Design review of the part built by this model. Coordinates are the model's own, in mm. A direction names the side the tool comes from. Coordinates: 2 decimals unless noted, no trailing zeros. Write each loop counter-clockwise with the first axis right and the second up, starting at its lowest first coordinate (ties: lowest second). Pieces come first, ordered by that corner, then holes.
Q1. Take a section at A-A (x = -18.5). Give the boundary of the cut face in (y, z), and give its area (3 significant figures).
Q2. Machinability: for faces 1 (the flat face through (-137.09, 3.13, 355.27)), 2 (the flat face through (-211.102, 3.131, -68.679)), 3 (the cylindrical face through (-120.638, 3.219, 125.96)), 4 (the flat face through (-138.21, 3.13, -107.53)), which of the approach directions +Z, -Z, +X, -X, +Y, -Y give a long, thin tool a straight path to every point of the face, cutting with its end or side? Answer none if there is none.
Q3. Insertion check: pin 1 (1.5 mm diameter, centred on y = 3, z = 326.5, fed in from -X); pin 2 (1 mm diameter, centred on y = 1.5, z = 330, fed in from +X); pin 3 (1.5 mm diameter, centred on x = 63.5, y = 4.5, fed in from +Z). Each pin has a flat end and moves straight along its axis. Give the tip position at first contact, or say it passes through.
Q4. Take a section at C-C (y = 3.75). State how many separate pieces and enclosed holes the cut face has, and give its area (3 significant figures).
Q5. For probe 1 along Z at (x, y) = (230, 2.75); probe 2 along Z at (x, y) = (-36, 5); probe 3 along Z at (x, y) = (159, 1), list the stretches that pass through material, from the lowest coordinate up.
Q6. Take a section at B-B (z = 196). Give the boundary of the cut face in (x, y).
Q7. Mouldability with a two-part tool opening along Z and no side actions: class faces 5 (the cylindrical face through (107.938, 3.219, 123.726)), 6 (the flat face through (-223.304, 3.131, -171.742)), 7 (the flat face through (138.213, 3.131, 357.218)) as pulls with the +Z half, pulls with the -Z half, needs draft (parallel to the pull), parting line crosses it, or undercut.
```python
from build123d import *

# Parameters (mm, degrees)
BOSS_EXTRUDE1_DEPTH     = 6.35
FILLET1_R               = 19.05
CUT_EXTRUDE1_DEPTH      = 503.879504709
SKETCH4_R               = 2.54
CUT_EXTRUDE2_DEPTH      = 503.879504709
SKETCH6_R               = 1.905
CUT_EXTRUDE3_DEPTH      = 503.879504709
MIRROR2_COPY_1_SKETCH_R = 2.54
MIRROR2_COPY_1_DEPTH    = 503.879504709
MIRROR2_COPY_2_SKETCH_R = 1.905
MIRROR2_COPY_2_DEPTH    = 503.879504709
FILLET2_R               = 12.7
SKETCH7_R               = 1.524
CUT_EXTRUDE4_DEPTH      = 503.879504709


with BuildPart() as part:
    # Sketch1 → Boss-Extrude1 (new body)
    with BuildSketch(Plane(origin=(0, 0, 0), x_dir=(1, 0, 0), z_dir=(0, 1, 0))):
        Polygon((-171.45, 0), (-258.780132361, 151.260226281), (-187.289735278, 192.535226281), (-92.039735278, 27.55738686), (92.039735278, 27.55738686), (187.289735278, 192.535226281), (258.780132361, 151.260226281), (171.45, 0), (171.45, -249.685226281), (258.780132361, -400.945452561), (187.289735278, -442.220452561), (92.039735278, -277.24261314), (-92.039735278, -277.24261314), (-187.289735278, -442.220452561), (-258.780132361, -400.945452561), (-171.45, -249.685226281), align=None)
    extrude(amount=BOSS_EXTRUDE1_DEPTH)

    # Fillet1
    fillet1_edges = [part.edges().sort_by_distance(p)[0] for p in [
        (-171.45, 3.175, 0),
        (-258.780132361, 3.175, -151.260226281),
        (-187.289735278, 3.175, -192.535226281),
        (-92.039735278, 3.175, -27.55738686),
        (92.039735278, 3.175, -27.55738686),
        (187.289735278, 3.175, -192.535226281),
        (258.780132361, 3.175, -151.260226281),
        (171.45, 3.175, 249.685226281),
        (258.780132361, 3.175, 400.945452561),
        (187.289735278, 3.175, 442.220452561),
        (92.039735278, 3.175, 277.24261314),
        (-92.039735278, 3.175, 277.24261314),
        (-187.289735278, 3.175, 442.220452561),
        (-258.780132361, 3.175, 400.945452561),
        (-171.45, 3.175, 249.685226281),
    ]]
    fillet(fillet1_edges, radius=FILLET1_R)

    # Sketch2 → Cut-Extrude1 (cut, through all)
    with BuildSketch(Plane(origin=(0, 6.35, 0), x_dir=(1, 0, 0), z_dir=(0, 1, 0))):
        with BuildLine():
            Line((-69.85, -74.04261314), (57.15, -74.04261314))
            ThreePointArc((57.15, -74.04261314), (107.95, -124.84261314), (57.15, -175.64261314))
            Line((57.15, -175.64261314), (-69.85, -175.64261314))
            ThreePointArc((-69.85, -175.64261314), (-120.65, -124.84261314), (-69.85, -74.04261314))
        make_face()
    cut_extrude1 = extrude(amount=-CUT_EXTRUDE1_DEPTH, mode=Mode.SUBTRACT)

    # Sketch4 → Cut-Extrude2 (cut, through all)
    with BuildSketch(Plane.XZ):
        with Locations(Location((198.392135104, -167.061146864, 0), (0, 0, 270))):
            Circle(SKETCH4_R)
        with Locations(Location((214.889919046, -157.536146864, 0), (0, 0, 270))):
            Circle(SKETCH4_R)
        with Locations(Location((231.387702988, -148.011146864, 0), (0, 0, 270))):
            Circle(SKETCH4_R)
        with Locations(Location((141.242135104, -68.074443212, 0), (0, 0, 90))):
            Circle(SKETCH4_R)
        with Locations(Location((174.237702988, -49.024443212, 0), (0, 0, 90))):
            Circle(SKETCH4_R)
        with Locations(Location((157.739919046, -58.549443212, 0), (0, 0, 90))):
            Circle(SKETCH4_R)
    cut_extrude2 = extrude(amount=-CUT_EXTRUDE2_DEPTH, mode=Mode.SUBTRACT)

    # Sketch6 → Cut-Extrude3 (cut, through all)
    with BuildSketch(Plane(origin=(0, 6.35, 0), x_dir=(1, 0, 0), z_dir=(0, 1, 0))):
        with Locations(Location((198.963220068, 100.740295038, 0), (0, 0, 270))):
            Circle(SKETCH6_R)
        with Locations(Location((185.951828097, 97.253903067, 0), (0, 0, 270))):
            Circle(SKETCH6_R)
        with Locations(Location((182.465436126, 110.265295038, 0), (0, 0, 270))):
            Circle(SKETCH6_R)
        with Locations(Location((195.476828097, 113.751687009, 0), (0, 0, 270))):
            Circle(SKETCH6_R)
    cut_extrude3 = extrude(amount=-CUT_EXTRUDE3_DEPTH, mode=Mode.SUBTRACT)

    # Mirror1: Cut-Extrude2, Cut-Extrude3 across plane
    add(cut_extrude2.mirror(Plane(origin=(0, 0, 0), x_dir=(0, 0, 1), z_dir=(1, 0, 0))), mode=Mode.SUBTRACT)
    add(cut_extrude3.mirror(Plane(origin=(0, 0, 0), x_dir=(0, 0, 1), z_dir=(1, 0, 0))), mode=Mode.SUBTRACT)

    # Mirror2: Cut-Extrude1, Cut-Extrude2, Cut-Extrude3 across plane
    add(cut_extrude1.mirror(Plane(origin=(0, 0, 124.84261314), x_dir=(1, 0, 0), z_dir=(0, 0, -1))), mode=Mode.SUBTRACT)
    add(cut_extrude2.mirror(Plane(origin=(0, 0, 124.84261314), x_dir=(1, 0, 0), z_dir=(0, 0, -1))), mode=Mode.SUBTRACT)
    add(cut_extrude3.mirror(Plane(origin=(0, 0, 124.84261314), x_dir=(1, 0, 0), z_dir=(0, 0, -1))), mode=Mode.SUBTRACT)

    # Mirror2 copy 1 sketch → Mirror2 copy 1 (cut, through all)
    with BuildSketch(Plane(origin=(0, 0, 249.685226281), x_dir=(-1, 0, 0), z_dir=(0, -1, 0))):
        with Locations(Location((198.392135104, -167.061146864, 0), (0, 0, 270))):
            Circle(MIRROR2_COPY_1_SKETCH_R)
        with Locations(Location((214.889919046, -157.536146864, 0), (0, 0, 270))):
            Circle(MIRROR2_COPY_1_SKETCH_R)
        with Locations(Location((231.387702988, -148.011146864, 0), (0, 0, 270))):
            Circle(MIRROR2_COPY_1_SKETCH_R)
        with Locations(Location((141.242135104, -68.074443212, 0), (0, 0, 90))):
            Circle(MIRROR2_COPY_1_SKETCH_R)
        with Locations(Location((174.237702988, -49.024443212, 0), (0, 0, 90))):
            Circle(MIRROR2_COPY_1_SKETCH_R)
        with Locations(Location((157.739919046, -58.549443212, 0), (0, 0, 90))):
            Circle(MIRROR2_COPY_1_SKETCH_R)
    extrude(amount=-MIRROR2_COPY_1_DEPTH, mode=Mode.SUBTRACT)

    # Mirror2 copy 2 sketch → Mirror2 copy 2 (cut, through all)
    with BuildSketch(Plane(origin=(0, 6.35, 249.685226281), x_dir=(-1, 0, 0), z_dir=(0, 1, 0))):
        with Locations(Location((198.963220068, 100.740295038, 0), (0, 0, 270))):
            Circle(MIRROR2_COPY_2_SKETCH_R)
        with Locations(Location((185.951828097, 97.253903067, 0), (0, 0, 270))):
            Circle(MIRROR2_COPY_2_SKETCH_R)
        with Locations(Location((182.465436126, 110.265295038, 0), (0, 0, 270))):
            Circle(MIRROR2_COPY_2_SKETCH_R)
        with Locations(Location((195.476828097, 113.751687009, 0), (0, 0, 270))):
            Circle(MIRROR2_COPY_2_SKETCH_R)
    extrude(amount=-MIRROR2_COPY_2_DEPTH, mode=Mode.SUBTRACT)

    # Fillet2
    fillet2_edges = [part.edges().sort_by_distance(p)[0] for p in [
        (171.45, 3.175, 0),
    ]]
    fillet(fillet2_edges, radius=FILLET2_R)

    # Sketch7 → Cut-Extrude4 (cut, through all)
    with BuildSketch(Plane(origin=(0, 6.35, 0), x_dir=(1, 0, 0), z_dir=(0, 1, 0))):
        with Locations(Location((-97.538996592, 14.85738686, 0), (0, 0, 270))):
            Circle(SKETCH7_R)
        with Locations(Location((-97.538996592, -6.73261314, 0), (0, 0, 270))):
            Circle(SKETCH7_R)
        with Locations(Location((-65.788996592, 14.85738686, 0), (0, 0, 270))):
            Circle(SKETCH7_R)
        with Locations(Location((-65.788996592, -6.73261314, 0), (0, 0, 270))):
            Circle(SKETCH7_R)
        with Locations(Location((97.538996592, -6.73261314, 0), (0, 0, 90))):
            Circle(SKETCH7_R)
        with Locations(Location((97.538996592, 14.85738686, 0), (0, 0, 90))):
            Circle(SKETCH7_R)
        with Locations(Location((65.788996592, 14.85738686, 0), (0, 0, 90))):
            Circle(SKETCH7_R)
        with Locations(Location((65.788996592, -6.73261314, 0), (0, 0, 90))):
            Circle(SKETCH7_R)
    extrude(amount=-CUT_EXTRUDE4_DEPTH, mode=Mode.SUBTRACT)


solid = part.part
```
Response:
1. outline: (0, -27.56) - (6.35, -27.56) - (6.35, 74.04) - (0, 74.04) - close; (0, 175.64) - (6.35, 175.64) - (6.35, 277.24) - (0, 277.24) - close
1. area: 1,290 mm2
2. face 1: +Z, +Y, -Y
2. face 2: -X, +Y, -Y
2. face 3: +Y, -Y
2. face 4: -Z, +Y, -Y
3. pin 1: stops at x = -216.23
3. pin 2: stops at x = 218.11
3. pin 3: stops at z = 277.24
4. separate pieces: 1
4. enclosed holes: 49
4. area: 138,000 mm2
5. probe 1: z = -167.88 to -150.14, -145.88 to -101.41, 351.1 to 395.57, 399.82 to 417.56
5. probe 2: z = -27.56 to 74.04, 175.64 to 277.24
5. probe 3: z = -143.54 to -60.75, -56.34 to 306.03, 310.44 to 393.22
6. outline: (-171.45, 0) - (171.45, 0) - (171.45, 6.35) - (-171.45, 6.35) - close
7. face 5: undercut
7. face 6: pulls with the -Z half
7. face 7: pulls with the +Z half
